```python
from build123d import *

# Parameters (mm, degrees)
BOSS_EXTRU_1_DEPTH           = 10
ESQUISSE3_R                  = 2.5
ENL_V_MAT_EXTRU_1_DEPTH      = 5
ENL_V_MAT_EXTRU_3_DEPTH      = 51.039984013
ENL_V_MAT_EXTRU_3_DEPTH_BACK = 51.039984013
ESQUISSE6_W                  = 20
ESQUISSE6_H                  = 12
ENL_V_MAT_EXTRU_4_DEPTH      = 6
ESQUISSE7_W                  = 20
ESQUISSE7_H                  = 12
BOSS_EXTRU_4_DEPTH           = 4


with BuildPart() as part:
    # Esquisse1 → Boss.-Extru.1 (new body)
    with BuildSketch(Plane(origin=(0, 0, 0), x_dir=(0, 0, -1), z_dir=(1, 0, 0))):
        with BuildLine():
            Line((0, 5), (-40, 5))
            ThreePointArc((-40, 5), (-45, 0), (-40, -5))
            Line((-40, -5), (0, -5))
            Line((0, -5), (20, -5))
            Line((20, -5), (20, -8))
            ThreePointArc((20, -8), (20.585786438, -9.414213562), (22, -10))
            Line((22, -10), (40, -10))
            Line((40, -10), (46.5, -10))
            ThreePointArc((46.5, -10), (47.560660172, -9.560660172), (48, -8.5))
            Line((48, -8.5), (48, 8.5))
            ThreePointArc((48, 8.5), (47.560660172, 9.560660172), (46.5, 10))
            Line((46.5, 10), (40, 10))
            Line((40, 10), (22, 10))
            ThreePointArc((22, 10), (20.585786438, 9.414213562), (20, 8))
            Line((20, 8), (20, 5))
            Line((20, 5), (0, 5))
        make_face()
    extrude(amount=BOSS_EXTRU_1_DEPTH)

    # Esquisse3 → Enlèv. mat.-Extru.1 (cut)
    with BuildSketch(Plane(origin=(10, 0, 0), x_dir=(0, 0, -1), z_dir=(1, 0, 0))):
        with Locations((-40, 0)):
            Circle(ESQUISSE3_R)
    extrude(amount=-ENL_V_MAT_EXTRU_1_DEPTH, mode=Mode.SUBTRACT)

    # Esquisse4 → Enlèv. mat.-Extru.3 (cut, two sides: drawn at the far end of the back side and taken through both)
    with BuildSketch(Plane(origin=(10, 0, 0), x_dir=(0, 0, -1), z_dir=(1, 0, 0)).offset(-ENL_V_MAT_EXTRU_3_DEPTH_BACK)):
        with BuildLine():
            ThreePointArc((35.333333333, 3.771236166), (46, 0), (35.333333333, -3.771236166))
            ThreePointArc((35.333333333, -3.771236166), (30, 0), (35.333333333, 3.771236166))
        make_face()
    extrude(amount=ENL_V_MAT_EXTRU_3_DEPTH + ENL_V_MAT_EXTRU_3_DEPTH_BACK, mode=Mode.SUBTRACT)

    # Esquisse6 → Enlèv. mat.-Extru.4 (cut)
    with BuildSketch(Plane(origin=(10, 0, 0), x_dir=(0, 0, -1), z_dir=(1, 0, 0))):
        with Locations((36, 0)):
            Rectangle(ESQUISSE6_W, ESQUISSE6_H)
    extrude(amount=-ENL_V_MAT_EXTRU_4_DEPTH, mode=Mode.SUBTRACT)

    # Esquisse7 → Boss.-Extru.4 (add)
    with BuildSketch(Plane(origin=(10, 0, 0), x_dir=(0, 0, -1), z_dir=(1, 0, 0))):
        with BuildLine():
            ThreePointArc((25.5, 8), (24.439339828, 7.560660172), (24, 6.5))
            Line((24, 6.5), (24, -6.5))
            ThreePointArc((24, -6.5), (24.439339828, -7.560660172), (25.5, -8))
            Line((25.5, -8), (46.5, -8))
            ThreePointArc((46.5, -8), (47.560660172, -7.560660172), (48, -6.5))
            Line((48, -6.5), (48, 6.5))
            ThreePointArc((48, 6.5), (47.560660172, 7.560660172), (46.5, 8))
            Line((46.5, 8), (25.5, 8))
        make_face()
        with Locations((36, 0)):
            Rectangle(ESQUISSE7_W, ESQUISSE7_H, mode=Mode.SUBTRACT)
    extrude(amount=BOSS_EXTRU_4_DEPTH)


solid = part.part
```
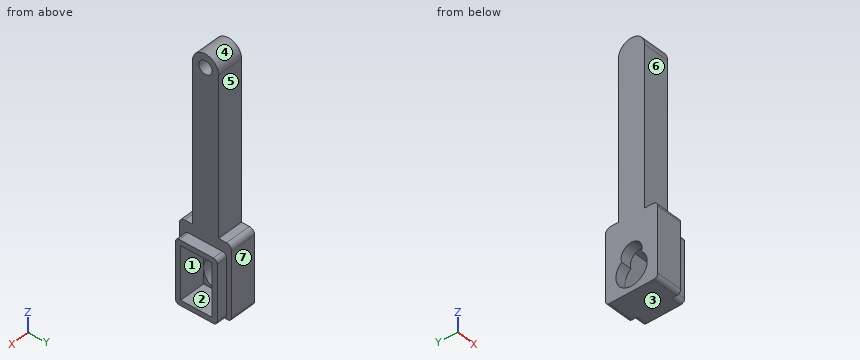
Geometry: final body of the model. Coordinates: model frame, mm. Face numbers are marked on the shaded views. A direction names the side the tool comes from. Coordinates: 2 decimals unless noted, no trailing zeros. Order: outer loops, then holes, each group sorted by start corner. A loop starts at its lowest first (then second) coordinate and runs counter-clockwise, first axis right, second up. Notation, with made-up numbers: M -3.75,25 L 2.25,25 A22 cw 2.25,57 Z; hole C -37.5,14.5 d7. An arc over 180 degrees is marked long. Answer in a Markdown table with one row per item. Add a question column.
Q1. Reachability of the marked faces 5, 6 and 7 from +Z, -Z, +X, -X, +Y, -Y: full face, straight path, thin tool, end or side. Return the list, or none.
Q2. Section query C-C on z = 16. Return the cut outline in (x, y), and give its area (3 significant figures).
Q3. Contact query for flat-ended pins moving along their axis: P1, Ø1.5, axis at x = 3.5, y = -7, coming from the +Z side; P2, Ø1.5, axis at x = 12.5, z = -35.5, coming from the -Y side; P3, Ø4, axis at y = 0, z = 40, coming from the +X side. Output: stop coordinate, or through.
Q4. Section query B-B on x = 2. Return the cut outline in (y, z), and give its area (3 significant figures).
Q5. Section query A-A on z = -34. Return the cut outline in (x, y), and give its area (3 significant figures).
Q6. Mould query, pull axis Z, two halves, no side actions, for the marked faces 1, 2, 3 and 4. Classes: released by +Z, released by -Z, zero draft, split by the parting line, or undercut.
Q7. Line query: L1, parallel to Y at x = 7.65, z = 40; L2, parallel to Z at x = 11.5, y = 4; L3, parallel to X at y = 1.75, z = -29.5. Output: solid intervals per line, ascending.
Completed:
| question | item | result |
|---|---|---|
| 1 | face 5 | +Z, +X, -X, +Y |
| 1 | face 6 | +Z, +X, -X, -Y |
| 1 | face 7 | +Z, -Z, +X, -X, +Y |
| 2 | outline | M 0,-5 L 10,-5 L 10,5 L 0,5 Z |
| 2 | area | 100 mm2 |
| 3 | P1 | stops at z = -20 |
| 3 | P2 | stops at y = -8 |
| 3 | P3 | stops at x = 5 |
| 4 | outline | M -10,-46.5 A1.5 ccw -8.5,-48 L 8.5,-48 A1.5 ccw 10,-46.5 L 10,-22 A2 ccw 8,-20 L 5,-20 L 5,40 A5 ccw -5,40 L -5,-20 L -8,-20 A2 ccw -10,-22 Z; hole M -3.77,-35.33 A6 ccw long 3.77,-35.33 A4 ccw long Z |
| 4 | area | 1,050 mm2 |
| 5 | outline | M 0,-10 L 10,-10 L 10,-8 L 14,-8 L 14,-6 L 4,-6 L 4,-4 L 0,-4 Z; M 0,4 L 4,4 L 4,6 L 14,6 L 14,8 L 10,8 L 10,10 L 0,10 Z |
| 5 | area | 112 mm2 |
| 6 | face 1 | undercut |
| 6 | face 2 | undercut |
| 6 | face 3 | released by -Z |
| 6 | face 4 | released by +Z |
| 7 | L1 | y = -5 to -2.5, 2.5 to 5 |
| 7 | L2 | z = -48 to -46, -26 to -24 |
| 7 | L3 | x = 0 to 4 |
